from build123d import *

# Parameters (mm, degrees)
SKETCH1_W           = 50
SKETCH1_H           = 75
BOSS_EXTRUDE1_DEPTH = 16
CUT_EXTRUDE1_DEPTH  = 36
SKETCH3_W           = 38
SKETCH3_H           = 24
BOSS_EXTRUDE4_DEPTH = 24
DRAFT2_ANGLE        = 10


with BuildPart() as part:
    # Sketch1 → Boss-Extrude1 (new, symmetric)
    with BuildSketch(Plane(origin=(0, 0, 0), x_dir=(1, 0, 0), z_dir=(0, 1, 0))):
        Rectangle(SKETCH1_W, SKETCH1_H)
    extrude(amount=BOSS_EXTRUDE1_DEPTH, both=True)

    # Sketch2 → Cut-Extrude1 (cut)
    with BuildSketch(Plane.XY.offset(37.5)):
        Polygon((0, 0), (-16, 16), (16, 16), align=None)
    extrude(amount=-CUT_EXTRUDE1_DEPTH, mode=Mode.SUBTRACT)

    # Sketch3 → Boss-Extrude4 (add)
    with BuildSketch(Plane(origin=(0, 16, 0), x_dir=(1, 0, 0), z_dir=(0, 1, 0))):
        with Locations((-6, 25.5)):
            Rectangle(SKETCH3_W, SKETCH3_H)
    extrude(amount=BOSS_EXTRUDE4_DEPTH)

    # Draft2
    draft2_faces = [part.faces().sort_by_distance(p)[0] for p in [
        (13, 28, -25.5),
        (-6, 28, -13.5),
    ]]
    draft(draft2_faces, Plane.ZX.offset(40), DRAFT2_ANGLE)


solid = part.part
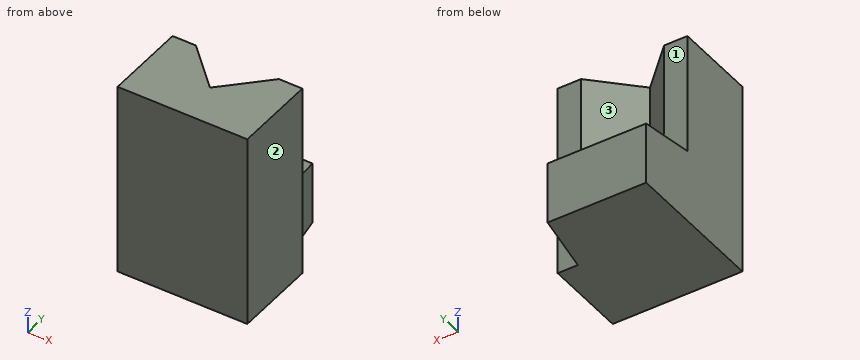
Here's how the part is built. I have some questions about the finished solid (model axes, mm). Face numbers are marked on the shaded views. Give positions to 0.01 mm unless a question says otherwise; leave off trailing zeros. Loops run counter-clockwise (first coordinate to the right, second up) from the corner with the lowest first, then second, coordinate; pieces in that order, holes last. Notation, with made-up numbers: (23.5, -8.75) -> (30.5, -8.75) arc R37 cw to (30.5, 30.25) -> close; hole circle Ø10 at (-15, -24.5). An arc over 180 degrees is marked (long way). Answer as a JSON object with one key per item and string values. Group by question number.
Item 1: Thinking about a two-plate mould opening in X: for the marked faces 1, 2 and 3, which applies, pulls with the +X half, pulls with the -X half, needs draft (parallel to the pull), parting line crosses it, or undercut?
Item 2: Imagine slicing it at C-C on z = 27.5. Write out the boundary of the cut face in (x, y), then the cut area to 3 significant figures.
Item 3: I need wall thicknesses on L1, parallel to Y at x = 14, z = -8.5; L2, parallel to Z at x = 1, y = 3.5; L3, parallel to Z at x = 3, y = 27. Which ranges of each line are inside material? Lowest first, please.
Item 4: Imagine slicing it at D-D on z = -5.5. Write out the boundary of the cut face in (x, y).
Item 5: Imagine slicing it at B-B on y = 1. Write out the boundary of the cut face in (x, z).
Item 6: Imagine slicing it at A-A on x = 1. Write out the boundary of the cut face in (y, z).
Item 7: Will this pin go through, and if not, where does the flat tip stop? pin 1 (2 mm diameter, centred on x = 0.5, z = 20, fed in from +Y).
Answer list:
{
 "1": {"face 1": "needs draft", "face 2": "pulls with the +X half", "face 3": "undercut"},
 "2": {"outline": "(-25, -16) -> (25, -16) -> (25, 16) -> (16, 16) -> (0, 0) -> (-16, 16) -> (-25, 16) -> close", "area": "1,340 mm2"},
 "3": {"L1": "y = -16 to 16", "L2": "z = -37.5 to 1.5", "L3": "z = -37.5 to -11.21"},
 "4": {"outline": "(-25, -16) -> (25, -16) -> (25, 16) -> (-25, 16) -> close"},
 "5": {"outline": "(-25, -37.5) -> (25, -37.5) -> (25, 37.5) -> (1, 37.5) -> (1, 1.5) -> (-1, 1.5) -> (-1, 37.5) -> (-25, 37.5) -> close"},
 "6": {"outline": "(-16, -37.5) -> (40, -37.5) -> (40, -13.5) -> (16, -9.27) -> (16, 1.5) -> (1, 1.5) -> (1, 37.5) -> (-16, 37.5) -> close"},
 "7": {"pin 1": "stops at y = 1.5"}
}
